CAD build for the part. Positions are in the model's coordinates, mm. Coordinates: 2 decimals unless noted, no trailing zeros. Loops run counter-clockwise (first coordinate to the right, second up) from the corner with the lowest first, then second, coordinate; pieces in that order, holes last. Notation, with made-up numbers: M 53,3 L 63,3 A26 cw 63,38 Z; hole C -5.75,51 d7. An arc over 180 degrees is marked long. Answer as a JSON object with one key per item and string values. Group by question number.
```python
from build123d import *

# Parameters (mm, degrees)
SKETCH2_W                        = 863.6
SKETCH2_H                        = 711.2
BOSS_EXTRUDE1_DEPTH              = 3.175
SKETCH3_W                        = 711.2
SKETCH3_H                        = 603.25
CUT_EXTRUDE2_DEPTH               = 1119.758454996
LPATTERN1_COUNT                  = 6
LPATTERN1_PITCH                  = 127
LPATTERN1_COUNT_DIR2             = 2
LPATTERN1_PITCH_DIR2             = 666.75
LPATTERN2_COUNT                  = 5
LPATTERN2_PITCH                  = 127
FILLET1_R                        = 6.35
F_21_64_0_32813_DIAMETER_HOLE1_D = 8.334502
LPATTERN4_COUNT                  = 2
LPATTERN4_PITCH                  = 736.6
LPATTERN4_COUNT_DIR2             = 2
LPATTERN4_PITCH_DIR2             = 628.65
F_21_64_0_32813_DIAMETER_HOLE2_D = 8.334502
LPATTERN5_COUNT                  = 5
LPATTERN5_PITCH                  = 127
LPATTERN5_COUNT_DIR2             = 2
LPATTERN5_PITCH_DIR2             = 628.65
F_21_64_0_32813_DIAMETER_HOLE3_D = 8.334502
LPATTERN6_COUNT                  = 4
LPATTERN6_PITCH                  = 127
LPATTERN6_COUNT_DIR2             = 2
LPATTERN6_PITCH_DIR2             = 736.6
LPATTERN7_COUNT                  = 5
LPATTERN7_PITCH                  = 127


with BuildPart() as part:
    # Sketch2 → Boss-Extrude1 (new body)
    with BuildSketch(Plane.XY):
        with Locations((431.8, 355.6)):
            Rectangle(SKETCH2_W, SKETCH2_H)
    extrude(amount=BOSS_EXTRUDE1_DEPTH)

    # Sketch3 → Cut-Extrude2 (cut, through all)
    with BuildSketch(Plane.XY.offset(3.175)):
        with Locations((457.2, 355.6)):
            Rectangle(SKETCH3_W, SKETCH3_H)
    extrude(amount=-CUT_EXTRUDE2_DEPTH, mode=Mode.SUBTRACT)

    # Sketch5 → CSK for 1/4 Flat Head Machine Screw1 (revolve, cut)
    with BuildSketch(Plane(origin=(114.3, 22.225, 3.175), x_dir=(0, -1, 0), z_dir=(1, 0, 0))):
        Polygon((0, 0), (0, 3.175), (3.57124, 3.175), (3.57124, 3.298865467), (6.4389, 0), align=None)
    csk_for_1_4_flat_head_machine_screw1 = revolve(axis=Axis((114.3, 22.225, 9.525), (0, 0, -1)), mode=Mode.SUBTRACT)

    # LPattern1: CSK for 1_4 Flat Head Machine Screw1 6 × 2
    with Locations(*[(i * LPATTERN1_PITCH, j * LPATTERN1_PITCH_DIR2, 0) for i in range(LPATTERN1_COUNT) for j in range(LPATTERN1_COUNT_DIR2) if (i, j) != (0, 0)]):
        add(csk_for_1_4_flat_head_machine_screw1, mode=Mode.SUBTRACT)

    # Sketch7 → CSK for 1/4 Flat Head Machine Screw2 (revolve, cut)
    with BuildSketch(Plane(origin=(841.375, 101.6, 3.175), x_dir=(0, -1, 0), z_dir=(1, 0, 0))):
        Polygon((0, 0), (0, 3.175), (3.57124, 3.175), (3.57124, 3.298865467), (6.4389, 0), align=None)
    csk_for_1_4_flat_head_machine_screw2 = revolve(axis=Axis((841.375, 101.6, 9.525), (0, 0, -1)), mode=Mode.SUBTRACT)

    # LPattern2: CSK for 1/4 Flat Head Machine Screw2 ×5
    with Locations(*[(0, i * LPATTERN2_PITCH, 0) for i in range(1, LPATTERN2_COUNT)]):
        add(csk_for_1_4_flat_head_machine_screw2, mode=Mode.SUBTRACT)

    # Fillet1
    fillet1_edges = [part.edges().sort_by_distance(p)[0] for p in [
        (101.6, 53.975, 1.5875),
        (101.6, 657.225, 1.5875),
        (812.8, 657.225, 1.5875),
        (812.8, 53.975, 1.5875),
    ]]
    fillet(fillet1_edges, radius=FILLET1_R)

    # 21/64 (0.32813) Diameter Hole1 (through all)
    with Locations(Plane.XY.offset(3.175)):
        with Locations((825.5, 41.275)):
            f_21_64_0_32813_diameter_hole1 = Hole(F_21_64_0_32813_DIAMETER_HOLE1_D / 2)

    # LPattern4: 21_64 _0.32813_ Diameter Hole1 2 × 2
    with Locations(*[(-i * LPATTERN4_PITCH, j * LPATTERN4_PITCH_DIR2, 0) for i in range(LPATTERN4_COUNT) for j in range(LPATTERN4_COUNT_DIR2) if (i, j) != (0, 0)]):
        add(f_21_64_0_32813_diameter_hole1, mode=Mode.SUBTRACT)

    # 21/64 (0.32813) Diameter Hole2 (through all)
    with Locations(Plane.XY.offset(3.175)):
        with Locations((685.8, 41.275)):
            f_21_64_0_32813_diameter_hole2 = Hole(F_21_64_0_32813_DIAMETER_HOLE2_D / 2)

    # LPattern5: 21_64 _0.32813_ Diameter Hole2 5 × 2
    with Locations(*[(-i * LPATTERN5_PITCH, j * LPATTERN5_PITCH_DIR2, 0) for i in range(LPATTERN5_COUNT) for j in range(LPATTERN5_COUNT_DIR2) if (i, j) != (0, 0)]):
        add(f_21_64_0_32813_diameter_hole2, mode=Mode.SUBTRACT)

    # 21/64 (0.32813) Diameter Hole3 (through all)
    with Locations(Plane.XY.offset(3.175)):
        with Locations((825.5, 165.1)):
            f_21_64_0_32813_diameter_hole3 = Hole(F_21_64_0_32813_DIAMETER_HOLE3_D / 2)

    # LPattern6: 21_64 _0.32813_ Diameter Hole3 4 × 2
    with Locations(*[(-j * LPATTERN6_PITCH_DIR2, i * LPATTERN6_PITCH, 0) for i in range(LPATTERN6_COUNT) for j in range(LPATTERN6_COUNT_DIR2) if (i, j) != (0, 0)]):
        add(f_21_64_0_32813_diameter_hole3, mode=Mode.SUBTRACT)

    # Sketch17 → CSK for #8 Flat Head Machine Screw1 (revolve, cut)
    with BuildSketch(Plane(origin=(88.9, 609.6, 3.175), x_dir=(0, -1, 0), z_dir=(1, 0, 0))):
        Polygon((0, 0), (0, 3.175), (2.2479, 3.175), (2.2479, 2.26450021), (4.2164, 0), align=None)
    csk_for_8_flat_head_machine_screw1 = revolve(axis=Axis((88.9, 609.6, 9.525), (0, 0, -1)), mode=Mode.SUBTRACT)

    # LPattern7: CSK for #8 Flat Head Machine Screw1 ×5
    with Locations(*[(0, -i * LPATTERN7_PITCH, 0) for i in range(1, LPATTERN7_COUNT)]):
        add(csk_for_8_flat_head_machine_screw1, mode=Mode.SUBTRACT)


solid = part.part
```
Item 1: Slice it at C-C, the plane z = 1.5. Count the separate pieces of the cut face and the enclosed holes in it, then the cut area to 3 significant figures.
Item 2: Slice it at A-A, the plane y = 591. Write the cut outline in (x, z) (3 decimals).
Item 3: Pin check, flat tip, straight feed: pin 1 (7.5 mm diameter, centred on x = 825.5, y = 546.1, fed in from +Z). Stop position of the tip, or through.
Item 4: Drill centre lines: L1, parallel to Y at x = 687, z = 0.25 (3 decimals); L2, parallel to Y at x = 685.8, z = 1.25 (3 decimals); L3, parallel to X at y = 111.5, z = 0.45. Where is each one in solid material? Low to high. Write a range as from..to.
Item 5: Slice it at B-B, the plane x = 528.5. Write the cut outline in (y, z) (3 decimals), then the cut area to 3 significant figures.
Computed:
{
 "1": {"separate pieces": "1", "enclosed holes": "45", "area": "183,000 mm2"},
 "2": {"outline": "M 0,0 L 101.6,0 L 101.6,3.175 L 0,3.175 Z; M 812.8,0 L 863.6,0 L 863.6,3.175 L 812.8,3.175 Z"},
 "3": {"pin 1": "through"},
 "4": {"L1": "0..37.284, 45.266..53.975, 657.225..665.934, 673.916..711.2", "L2": "0..37.108, 45.442..53.975, 657.225..665.758, 674.092..711.2", "L3": "0..101.6, 812.8..863.6"},
 "5": {"outline": "M 0,0 L 53.975,0 L 53.975,3.175 L 0,3.175 Z; M 657.225,0 L 711.2,0 L 711.2,3.175 L 657.225,3.175 Z", "area": "343 mm2"}
}
